Model file for the job. Use its own axes, mm. A direction names the side the tool comes from. Round coordinates to 2 decimals unless told otherwise and drop trailing zeros. Loops run counter-clockwise (first coordinate to the right, second up) from the corner with the lowest first, then second, coordinate; pieces in that order, holes last.
Autodesk Inventor part; units mm, degrees
ref_plane "YZ Plane" through (0, 0, 0) normal (1, 0, 0) x (0, 1, 0)
ref_plane "XZ Plane" through (0, 0, 0) normal (0, 1, 0) x (-1, 0, 0)
ref_plane "XY Plane" through (0, 0, 0) normal (0, 0, 1) x (1, 0, 0)
sketch "Sketch1" plane through (0, 0, 0) normal (0, 0, 1) x (1, 0, 0)
  circle A0 centre (0, 0) radius 4
  circle A1 centre (0, 0) radius 10
  circle A2 centre (-6.9282, -4) radius 1.0065
  circle A3 centre (6.9282, -4) radius 1.0065
  circle A4 centre (0, 8) radius 1.0065
  dimension "d0" = 8
  dimension "d1" = 20
extrude "Extrusion1" add sketch "Sketch1" along normal blind 5
sketch "Sketch2" plane through (0, 0, 5) normal (0, 0, 1) x (1, 0, 0)
  circle A0 centre (0, 0) radius 4
  circle A1 centre (0, 0) radius 10
  line L0 (3.9976, 0.1396) -> (13.5917, 0.4746)
  line L1 (7.2069, 11.5335) -> (2.1197, 3.3922)
  line L2 (3.9976, 0.1396) -> (6.6264, 0.2314)
  line L3 (9.9939, 0.349) -> (5.2992, 8.4805)
  line L4 (9.9939, 0.349) -> (3.9976, 0.1396)
  line L5 (2.1197, 3.3922) -> (5.2992, 8.4805)
  arc A2 (3.9976, 0.1396) -> (2.1197, 3.3922) centre (0, 0) ccw
  arc A3 (9.9939, 0.349) -> (5.2992, 8.4805) centre (0, 0) ccw
extrude "Extrusion2" cut sketch "Sketch2" against normal blind 5 contours A0 L1 L3 L0 | A1 L3
pattern_circular "Circular Pattern1" count 3 over 360 about axis through (0, 0, 0) along (0, 0, 1) of "Extrusion2"
sketch "Sketch3" plane through (0, 0, 5) normal (0, 0, 1) x (1, 0, 0)
  arc A0 (-9.9939, 0.349) -> (-4.6947, -8.8295) centre (0, 0) ccw
  circle A1 centre (0, 0) radius 5
  dimension "d9" = 10
extrude "Extrusion3" add sketch "Sketch3" against normal blind 5
sketch "Sketch4" plane through (0, 0, 5) normal (0, 0, 1) x (1, 0, 0)
  circle A0 centre (6.9282, -4) radius 1.0065
  circle A1 centre (0, 8) radius 1.0065
  circle A2 centre (-6.9282, -4) radius 1.0065
  circle A3 centre (-6.9282, -4) radius 1.6
  circle A4 centre (6.9282, -4) radius 1.6
  circle A5 centre (0, 8) radius 1.6
  dimension "d12" = 3.2
  dimension "d13" = 3.2
  dimension "d14" = 3.2
extrude "Extrusion4" cut sketch "Sketch4" against normal blind 3
sketch "Sketch5" plane through (0, 0, 5) normal (0, 0, 1) x (1, 0, 0)
  arc A0 (-9.9939, 0.349) -> (-4.6947, -8.8295) centre (0, 0) ccw
  circle A1 centre (0, 0) radius 2
  dimension "d17" = 4
extrude "Extrusion5" add sketch "Sketch5" along normal blind 8
sketch "Sketch6" plane through (0, 0, 13) normal (0, 0, 1) x (1, 0, 0)
  circle A0 centre (0, 0) radius 2
  circle A1 centre (0, 0) radius 1.9
  dimension "d20" = 3.8
extrude "Extrusion6" add sketch "Sketch6" along normal blind 0.4 contours A1
sketch "Sketch7" plane through (0, 0, 13.4) normal (0, 0, 1) x (1, 0, 0)
  circle A0 centre (0, 0) radius 1.9
  circle A1 centre (0, 0) radius 2
  dimension "d23" = 4
extrude "Extrusion7" add sketch "Sketch7" along normal blind 10 contours A0 | A1
thread "Thread1"
chamfer "Chamfer1" distance 0.4 angle 45 1 edges at (-2, 0, 23.4)
sketch "Sketch8" plane through (0, 0, 0) normal (0, 1, 0) x (-1, 0, 0)
  line L0 (-1.6, 23.4) -> (1.6, 23.4)
  line L1 (0, 25.3241) -> (0, 15.4)
  line L2 (0, 15.4) -> (4.0898, 15.4)
  spline S0 degree 3 poles (0, 25.3241) (0.1432, 25.2864) (2.524, 24.659) (3.9837, 20.08) (4.062, 16.6285) (4.0898, 15.4) knots 0 0 0 0 0.044151 0.734206 1.11559 1.11559 1.11559 1.11559
  point P0 (0, 0)
  point P1 (0.4244, 25.2023)
  point P2 (3.8385, 19.2055)
  dimension "d32" = 8
  dimension "d33" = 9.9241
revolve "Revolution1" add sketch "Sketch8" angle 360 about axis through (0, 0, 25.3241) along (0, 0, -1)
sketch "Sketch9" plane through (0, 0, 0) normal (1, 0, 0) x (0, 1, 0)
  line L0 (-4.0898, 15.4) -> (4.0898, 15.4)
  line L1 (0, 15.4) -> (0, 21.1198)
  circle A0 centre (0, 21.1198) radius 0.75
  point P0 (0, 0)
  dimension "d34" = 1.5
extrude "Extrusion8" cut sketch "Sketch9" against normal mid plane 20
equation "\"d13\" = d12"
equation "\"d14\" = d13"
properties part number "HK 2830 1100 prop adapter"
Q1. Pull direction X, two halves, no side cores. Call faces 1 (the face through (-3.956, 6.331, 2.535)), 2 (the face through (-3.505, -6.591, 2.535)), 3 (the face through (-1.9, -0.08, 13.2)): pulls with the +X half, pulls with the -X half, needs draft (parallel to the pull), parting line crosses it, or undercut.
Q2. Slice it at C-C on z = 4.25. Give the cut face in (x, y), plus the area to 3 significant figures.
Q3. Tool access for faces 4 (the face through (0, 2, 14)), 5 (the face through (0.051, -0.163, 20.388)), 6 (the face through (0, 10, 2)), 7 (the face through (4, 6.4, 2.5)), 8 (the face through (-1, 9, 2)): list every direction of +Z, -Z, +X, -X, +Y, -Y with a clear straight run to the whole face (end or side of a thin tool).
Q4. Probe line 1 (Y direction, x = 0, z = 0.75); line 2 (Y direction, x = 0, z = 4.1); line 3 (Z direction, x = -2.25, y = 0.25). List the from-to ranges inside material, lowest first.
Q5. Slice it at B-B on y = 8. Give the cut face in (x, z).
Q6. Slice it at A-A on x = 7.5. Give the cut face in (y, z).
Q7. Flat gauge pins, fed straight in: P1, Ø2.5, axis at x = -6.93, y = -4, coming from the +Z side; P2, Ø5, axis at x = 6.93, y = -4, coming from the +Z side; P3, Ø4, axis at x = 5.5, y = 3.5, coming from the -Z side; P4, Ø5.5, axis at x = -4, y = -3.5, coming from the +Z side. Where does each tip first touch, or does it go through?
Q8. Slice it at D-D on x = 0.5. State how many separate pieces and enclosed holes the cut face has, plus the area to 3 significant figures.
Reply:
1. face 1: pulls with the -X half
1. face 2: undercut
1. face 3: parting line crosses it
2. outline: (-9.99, 0.35) arc R10 ccw to (-4.69, -8.83) - (-2.35, -4.41) arc R5 ccw to (2.35, -4.41) - (4.69, -8.83) arc R10 ccw to (9.99, 0.35) - (5, 0.17) arc R5 ccw to (2.65, 4.24) - (5.3, 8.48) arc R10 ccw to (-5.3, 8.48) - (-2.65, 4.24) arc R5 ccw to (-5, 0.17) - close; hole circle Ø3.2 at (-6.93, -4); hole circle Ø3.2 at (0, 8); hole circle Ø3.2 at (6.93, -4)
2. area: 180 mm2
3. face 4: none
3. face 5: +X, -X
3. face 6: +Z, -Z, +Y
3. face 7: +Z, -Z, +X
3. face 8: +Z
4. line 1: y = -5 to 6.99, 9.01 to 10
4. line 2: y = -5 to 6.4, 9.6 to 10
4. line 3: z = 0 to 5, 15.4 to 20.41, 21.83 to 23.77
5. outline: (-5, 0) - (-1.01, 0) - (-1.01, 2) - (-1.6, 2) - (-1.6, 5) - (-5, 5) - close; (1.01, 0) - (5, 0) - (5, 5) - (1.6, 5) - (1.6, 2) - (1.01, 2) - close
6. outline: (-6.61, 0) - (-4.83, 0) - (-4.83, 2) - (-5.49, 2) - (-5.49, 5) - (-6.61, 5) - close; (-3.17, 0) - (0.26, 0) - (0.26, 5) - (-2.51, 5) - (-2.51, 2) - (-3.17, 2) - close
7. P1: stops at z = 2
7. P2: stops at z = 5
7. P3: stops at z = 0
7. P4: stops at z = 23.3
8. separate pieces: 2
8. enclosed holes: 1
8. area: 164 mm2
